Verification items for the finished model (mm, model axes). Face numbers are marked on the shaded views. Coordinates: 2 decimals unless noted, no trailing zeros. Order: outer loops, then holes, each group sorted by start corner. A loop starts at its lowest first (then second) coordinate and runs counter-clockwise, first axis right, second up. Notation, with made-up numbers: (1.5, 59.25) -> (16.5, 59.25) arc R23 cw to (16.5, 83.25) -> close; hole circle Ø2 at (84.25, -16.75). An arc over 180 degrees is marked (long way). Use CSV: the item, a comma, the result in double quotes. Start each with the question number.
1) Go/stop test with flat-tipped pins: pin 1 (1.5 mm diameter, centred on x = -5, z = 6, fed in from -Y); pin 2 (1 mm diameter, centred on x = -5.5, z = 9, fed in from -Y); pin 3 (1.2 mm diameter, centred on x = 0, z = 0, fed in from +Y). Record where each tip stops, or that it passes through.
2) Sectioned sample at A-A on x = -1. Record the boundary of the cut face in (y, z) (3 decimals), then the cut area to 3 significant figures.
3) Sectioned sample at C-C on z = -6.75. Record the boundary of the cut face in (x, y), then the cut area to 3 significant figures.
4) Sectioned sample at D-D on z = -2.25. Record the boundary of the cut face in (x, y).
5) Scan lines: line 1 along Z through (x, y) = (5.25, -4.25) (3 decimals); line 2 along Y through (x, z) = (5, -1.25); line 3 along Y through (x, z) = (-4, 7). Record each from-to range of solid material in increasing order.
6) Release check for a two-part mould opening along X. For the marked faces 1, 2 and 3 record: released by +X, released by -X, zero draft, split by the parting line, or undercut.
7) Sectioned sample at B-B on y = -3.5. Give the number of separate pieces and of enclosed holes in the cut face, then the cut area to 3 significant figures.
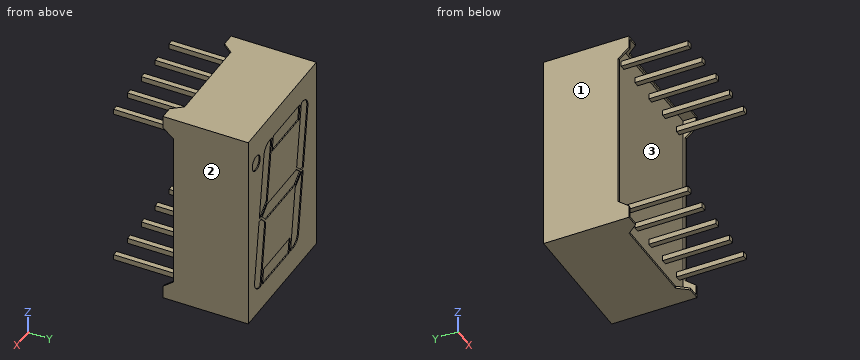
from build123d import *

# Parameters (mm, degrees)
CROQUIS1_W              = 12.5
CROQUIS1_H              = 19
SALIENTE_EXTRUIR1_DEPTH = 8
CROQUIS4_W              = 12.1
CROQUIS4_H              = 18.6
CORTAR_EXTRUIR3_DEPTH   = 1
CORTAR_EXTRUIR1_DEPTH   = 18.621010187
CORTAR_EXTRUIR2_DEPTH   = 22.542109925
CROQUIS5_W              = 12.1
CROQUIS5_H              = 18.6
CORTAR_EXTRUIR4_DEPTH   = 0.2
CROQUIS6_W              = 0.51
CROQUIS6_H              = 0.51
SALIENTE_EXTRUIR2_DEPTH = 6.3
CROQUIS7_R              = 0.725
CORTAR_EXTRUIR5_DEPTH   = 0.1


with BuildPart() as part:
    # Croquis1 → Saliente-Extruir1 (new body)
    with BuildSketch(Plane(origin=(0, 0, 0), x_dir=(1, 0, 0), z_dir=(0, 1, 0))):
        Rectangle(CROQUIS1_W, CROQUIS1_H)
    extrude(amount=SALIENTE_EXTRUIR1_DEPTH)

    # Croquis4 → Cortar-Extruir3 (cut)
    with BuildSketch(Plane(origin=(0, 0, 0), x_dir=(1, 0, 0), z_dir=(0, 1, 0))):
        Rectangle(CROQUIS4_W, CROQUIS4_H)
    extrude(amount=CORTAR_EXTRUIR3_DEPTH, mode=Mode.SUBTRACT)

    # Croquis2 → Cortar-Extruir1 (cut, through all)
    with BuildSketch(Plane(origin=(6.25, 0, 0), x_dir=(0, 0, -1), z_dir=(1, 0, 0))):
        Polygon((-8.3, 0), (0, 0), (0, 1), (-7.5, 1), align=None)
        Polygon((0, 1), (0, 0), (8.3, 0), (7.5, 1), align=None)
    extrude(amount=-CORTAR_EXTRUIR1_DEPTH, mode=Mode.SUBTRACT)

    # Croquis3 → Cortar-Extruir2 (cut, through all)
    with BuildSketch(Plane.XY.offset(9.5)):
        Polygon((0, 1), (0, 0), (5.05, 0), (4.25, 1), align=None)
        Polygon((-5.05, 0), (0, 0), (0, 1), (-4.25, 1), align=None)
    extrude(amount=-CORTAR_EXTRUIR2_DEPTH, mode=Mode.SUBTRACT)

    # Croquis5 → Cortar-Extruir4 (cut)
    with BuildSketch(Plane.XZ.offset(-1)):
        Rectangle(CROQUIS5_W, CROQUIS5_H)
    extrude(amount=-CORTAR_EXTRUIR4_DEPTH, mode=Mode.SUBTRACT)

    # Croquis6 → Saliente-Extruir2 (add)
    with BuildSketch(Plane.XZ.offset(-1.2)):
        with Locations((5.08, 7.62)):
            Rectangle(CROQUIS6_W, CROQUIS6_H)
        with Locations((-5.08, 7.62)):
            Rectangle(CROQUIS6_W, CROQUIS6_H)
        with Locations((-2.54, 7.62)):
            Rectangle(CROQUIS6_W, CROQUIS6_H)
        with Locations((0, 7.62)):
            Rectangle(CROQUIS6_W, CROQUIS6_H)
        with Locations((2.54, 7.62)):
            Rectangle(CROQUIS6_W, CROQUIS6_H)
        with Locations((5.08, -7.62)):
            Rectangle(CROQUIS6_W, CROQUIS6_H)
        with Locations((2.54, -7.62)):
            Rectangle(CROQUIS6_W, CROQUIS6_H)
        with Locations((0, -7.62)):
            Rectangle(CROQUIS6_W, CROQUIS6_H)
        with Locations((-2.54, -7.62)):
            Rectangle(CROQUIS6_W, CROQUIS6_H)
        with Locations((-5.08, -7.62)):
            Rectangle(CROQUIS6_W, CROQUIS6_H)
    extrude(amount=SALIENTE_EXTRUIR2_DEPTH)

    # Croquis7 → Cortar-Extruir5 (cut)
    with BuildSketch(Plane(origin=(0, 8, 0), x_dir=(1, 0, 0), z_dir=(0, 1, 0))):
        with BuildLine():
            Line((5.08455374, 5.950418058), (4.266083352, 0.125))
            Line((4.266083352, 0.125), (3.866083352, 0.125))
            Line((3.866083352, 0.125), (3.037577222, 0.989725951))
            Line((3.037577222, 0.989725951), (3.894601803, 7.089551363))
            Line((3.894601803, 7.089551363), (4.094280079, 7.089551363))
            ThreePointArc((4.094280079, 7.089551363), (4.848976476, 6.745625556), (5.08455374, 5.950418058))
        make_face()
        with BuildLine():
            Line((1.9, -7.106917481), (2.380677984, -7.106917481))
            ThreePointArc((2.380677984, -7.106917481), (3.036752178, -6.861613878), (3.370951645, -6.246050786))
            Line((3.370951645, -6.246050786), (4.230255889, -0.13))
            Line((4.230255889, -0.13), (3.866081115, -0.13))
            Line((3.866081115, -0.13), (2.753310906, -1.033523948))
            Line((2.753310906, -1.033523948), (1.9, -7.106917481))
        make_face()
        Polygon((0, 0.725), (-2.399616736, 0.725), (-2.604044024, -0.73), (0, -0.73), (2.795955976, -0.73), (3.000383264, 0.725), align=None)
        Polygon((1.853724789, -5.656917481), (-3.043819744, -5.656917481), (-3.247544533, -7.106917481), (1.65, -7.106917481), align=None)
        with BuildLine():
            ThreePointArc((-3.699678276, -7.106917481), (-4.454374673, -6.762991674), (-4.689951937, -5.967784176))
            Line((-4.689951937, -5.967784176), (-3.869744111, -0.13))
            Line((-3.869744111, -0.13), (-3.476909246, -0.13))
            Line((-3.476909246, -0.13), (-2.633262018, -0.937957469))
            Line((-2.633262018, -0.937957469), (-3.5, -7.106917481))
            Line((-3.5, -7.106917481), (-3.699678276, -7.106917481))
        make_face()
        with BuildLine():
            ThreePointArc((-2.976349842, 6.228684668), (-2.642150375, 6.84424776), (-1.986076181, 7.089551363))
            Line((-1.986076181, 7.089551363), (-1.505398197, 7.089551363))
            Line((-1.505398197, 7.089551363), (-2.358391548, 1.018418011))
            Line((-2.358391548, 1.018418011), (-3.549623917, 0.125))
            Line((-3.549623917, 0.125), (-3.833916648, 0.125))
            Line((-3.833916648, 0.125), (-2.976349842, 6.228684668))
        make_face()
        Polygon((-2.399616736, 0.725), (-2.604044024, -0.73), (-3.366290182, 0), align=None)
        Polygon((3.000383264, 0.725), (3.69501599, 0), (2.795955976, -0.73), align=None)
        with Locations(Location((4.787756453, -6.368008077, 0), (0, 0, 270))):
            Circle(CROQUIS7_R)
        Polygon((-1.25294273, 7.089551363), (-1.456667518, 5.639551363), (0, 5.639551363), (3.441812575, 5.639551363), (3.645537364, 7.089551363), (0, 7.089551363), align=None)
    extrude(amount=-CORTAR_EXTRUIR5_DEPTH, mode=Mode.SUBTRACT)


solid = part.part
Answers follow:
1,pin 1,"stops at y = 1.2"
1,pin 2,"stops at y = 0"
1,pin 3,"stops at y = 7.9"
2,outline,"(1, -9.5) -> (8, -9.5) -> (8, -7.09) -> (7.9, -7.09) -> (7.9, -5.64) -> (8, -5.64) -> (8, -0.725) -> (7.9, -0.725) -> (7.9, 0.73) -> (8, 0.73) -> (8, 5.657) -> (7.9, 5.657) -> (7.9, 7.107) -> (8, 7.107) -> (8, 9.5) -> (1, 9.5) -> (1, 9.3) -> (1.2, 9.3) -> (1.2, -9.3) -> (1, -9.3) -> close"
2,area,"129 mm²"
3,outline,"(-6.25, 1) -> (-6.05, 1) -> (-6.05, 1.2) -> (6.05, 1.2) -> (6.05, 1) -> (6.25, 1) -> (6.25, 8) -> (4.85, 8) -> (4.85, 7.9) -> (3.85, 7.9) -> (3.85, 8) -> (3.6, 8) -> (3.6, 7.9) -> (-1.3, 7.9) -> (-1.3, 8) -> (-1.55, 8) -> (-1.55, 7.9) -> (-2.74, 7.9) -> (-2.74, 8) -> (-6.25, 8) -> close"
3,area,"84.4 mm²"
4,outline,"(-6.25, 1) -> (-6.05, 1) -> (-6.05, 1.2) -> (6.05, 1.2) -> (6.05, 1) -> (6.25, 1) -> (6.25, 8) -> (4.56, 8) -> (4.56, 7.9) -> (3.21, 7.9) -> (3.21, 8) -> (-2.19, 8) -> (-2.19, 7.9) -> (-3.54, 7.9) -> (-3.54, 8) -> (-6.25, 8) -> close"
5,line 1,"z = -7.875 to -7.365, 7.365 to 7.875"
5,line 2,"y = 1.2 to 8"
5,line 3,"y = 1.2 to 7.9"
6,face 1,"released by -X"
6,face 2,"released by +X"
6,face 3,"undercut"
7,separate pieces,"10"
7,enclosed holes,"0"
7,area,"2.60 mm²"
